For this review, take the finished solid that the model builds, in its own axes (mm). Coordinates: 2 decimals unless noted, no trailing zeros. Order: outer loops, then holes, each group sorted by start corner. A loop starts at its lowest first (then second) coordinate and runs counter-clockwise, first axis right, second up.
from build123d import *

# Parameters (mm, degrees)
F0_R     = 12.7
F0_R_2   = 44.45
F1_DEPTH = 6.35


# Not quite as in the source:
# - a length typed as a fraction of an inch, garbled in the dataset ("3 / 203.2 mm" for 3/8 in), is restored


with BuildPart() as f1:
    # F0 (on Right) → F1 (new body)
    with BuildSketch(Plane.YZ):
        with BuildLine():
            Line((44.8562400312, 44.8719321083), (44.6357637569, 45.1652365635))
            ThreePointArc((44.6357637569, 45.1652365635), (-0.039236718, 63.4999878778), (-44.6915449582, 45.1100411133))
            ThreePointArc((-44.6915449582, 45.1100411133), (-58.4915893115, 33.8212553621), (-76.2, 31.75))
            ThreePointArc((-76.2, 31.75), (-107.95, 0), (-76.2, -31.75))
            ThreePointArc((-76.2, -31.75), (-58.4915893115, -33.8212553621), (-44.6915449582, -45.1100411133))
            ThreePointArc((-44.6915449582, -45.1100411133), (0, -63.5), (44.6915449582, -45.1100411133))
            ThreePointArc((44.6915449582, -45.1100411133), (58.4915893115, -33.8212553621), (76.2, -31.75))
            ThreePointArc((76.2, -31.75), (107.95, 0), (76.2, 31.75))
            ThreePointArc((76.2, 31.75), (58.6249913094, 33.7650494266), (44.8562400312, 44.8719321083))
        make_face()
        with Locations((-76.2, 0)):
            Circle(F0_R, mode=Mode.SUBTRACT)
        Circle(F0_R_2, mode=Mode.SUBTRACT)
        with Locations((76.2, 0)):
            Circle(F0_R, mode=Mode.SUBTRACT)
    extrude(amount=F1_DEPTH)


solid = f1.part
1. The part is to be moulded in two halves that separate along Z. For faces 1 (the face through (0, 46, 1)), 2 (the face through (3.131, 42.397, 13.352)), 3 (the face through (3.131, -107.942, 0.698)), say which applies: +Z half, -Z half, draft (parallel to the pull), parting line (faces both ways), or undercut.
Answer below:
face 1: draft
face 2: undercut
face 3: parting line
2. Take a section at C-C, the plane z = 0. Give the boundary of the cut face in (x, y).
Answer below:
outline: (0, -107.95) - (6.35, -107.95) - (6.35, -88.9) - (0, -88.9) - close; (0, -63.5) - (6.35, -63.5) - (6.35, -44.45) - (0, -44.45) - close; (0, 44.45) - (6.35, 44.45) - (6.35, 63.5) - (0, 63.5) - close; (0, 88.9) - (6.35, 88.9) - (6.35, 107.95) - (0, 107.95) - close
3. Take a section at B-B, the plane x = 3.5. Give the boundary of the cut face in (y, z).
Answer below:
outline: (-76.2, -31.75) arc R31.75 cw to (-44.69, -45.11) arc R63.5 ccw to (44.69, -45.11) arc R31.75 cw to (76.2, -31.75) arc R31.75 ccw to (76.2, 31.75) arc R31.75 cw to (44.86, 44.87) - (44.64, 45.17) arc R63.5 ccw to (-44.69, 45.11) arc R31.75 cw to (-76.2, 31.75) arc R31.75 ccw to start; hole circle Ø25.4 at (-76.2, 0); hole circle Ø88.9 at (0, 0); hole circle Ø25.4 at (76.2, 0)
4. Clearance check with flat-ended pins moving along their axes: pin 1 Ø3 at (x, z) = (3.5, 40.5) entering from +Y; pin 2 Ø2 at (x, y) = (5, 70.5) entering from -Z. State where each tip first meets the part, or that it passes through.
Answer below:
pin 1: stops at y = 50.16
pin 2: stops at z = -31.33
5. Take a section at A-A, the plane y = 0. Give the boundary of the cut face in (x, z), plus the area to 3 significant figures.
Answer below:
outline: (0, -63.5) - (6.35, -63.5) - (6.35, -44.45) - (0, -44.45) - close; (0, 44.45) - (6.35, 44.45) - (6.35, 63.5) - (0, 63.5) - close
area: 242 mm2
6. Take a section at D-D, the plane z = 15. Give the boundary of the cut face in (x, y), plus the area to 3 significant figures.
Answer below:
outline: (0, -104.18) - (6.35, -104.18) - (6.35, -41.84) - (0, -41.84) - close; (0, 41.84) - (6.35, 41.84) - (6.35, 104.18) - (0, 104.18) - close
area: 792 mm2
7. To check wall thickness, follow L1, parallel to Y at x = 0.5, z = 1; L2, parallel to Z at x = 4.5, y = 76.2; L3, parallel to Z at x = 2, y = 0. State the ranges of each line that lie inside material, in increasing order.
Answer below:
L1: y = -107.93 to -88.86, -63.54 to -44.44, 44.44 to 63.54, 88.86 to 107.93
L2: z = -31.75 to -12.7, 12.7 to 31.75
L3: z = -63.5 to -44.45, 44.45 to 63.5
